Autodesk Inventor part; units mm, degrees
ref_plane "YZ Plane" through (0, 0, 0) normal (1, 0, 0) x (0, 1, 0)
ref_plane "XZ Plane" through (0, 0, 0) normal (0, 1, 0) x (-1, 0, 0)
ref_plane "XY Plane" through (0, 0, 0) normal (0, 0, 1) x (1, 0, 0)
sketch "Boceto1" plane through (0, 0, 0) normal (1, 0, 0) x (0, 1, 0)
  line L0 (25, 5.601225) -> (19, 5.601225)
  line L1 (19, 5.601225) -> (19, -18.398775)
  line L2 (19, -18.398775) -> (15, -18.398775)
  line L3 (15, -18.398775) -> (15, -80.798775)
  line L4 (15, -80.798775) -> (45, -80.798775)
  line L5 (45, -80.798775) -> (45, -68.598775)
  line L6 (45, -68.598775) -> (20, -68.598775)
  line L7 (20, -68.598775) -> (20, -24.398775)
  line L8 (20, -24.398775) -> (25, -24.398775)
  line L9 (25, -24.398775) -> (25, 5.601225)
  line L10 (0, 0) -> (0, 11.507163) construction
  line L11 (-25, 5.601225) -> (-19, 5.601225)
  line L12 (-19, 5.601225) -> (-19, -18.398775)
  line L13 (-19, -18.398775) -> (-15, -18.398775)
  line L14 (-15, -18.398775) -> (-15, -80.798775)
  line L15 (-15, -80.798775) -> (-45, -80.798775)
  line L16 (-45, -80.798775) -> (-45, -68.598775)
  line L17 (-45, -68.598775) -> (-20, -68.598775)
  line L18 (-20, -68.598775) -> (-20, -24.398775)
  line L19 (-20, -24.398775) -> (-25, -24.398775)
  line L20 (-25, -24.398775) -> (-25, 5.601225)
  dimension "d0" = 30
  dimension "d1" = 40
  dimension "d2" = 90
  dimension "d3" = 38
  dimension "d4" = 50
  dimension "d5" = 24
  dimension "d6" = 6
  dimension "d7" = 44.2
  dimension "d8" = 12.2
sketch "Boceto1 outline for Revolución1" plane through (0, 0, 0) normal (1, 0, 0) x (0, 1, 0)
  line L0 (-25, 5.601225) -> (-25, -24.398775)
  line L1 (-19, 5.601225) -> (-25, 5.601225)
  line L2 (-19, -18.398775) -> (-19, 5.601225)
  line L3 (-15, -18.398775) -> (-19, -18.398775)
  line L4 (-15, -80.798775) -> (-15, -18.398775)
  line L5 (-45, -80.798775) -> (-15, -80.798775)
  line L6 (-45, -68.598775) -> (-45, -80.798775)
  line L7 (-20, -68.598775) -> (-45, -68.598775)
  line L8 (-20, -24.398775) -> (-20, -68.598775)
  line L9 (-25, -24.398775) -> (-20, -24.398775)
  line L10 (25, 5.601225) -> (19, 5.601225)
  line L11 (25, -24.398775) -> (25, 5.601225)
  line L12 (20, -24.398775) -> (25, -24.398775)
  line L13 (20, -68.598775) -> (20, -24.398775)
  line L14 (45, -68.598775) -> (20, -68.598775)
  line L15 (45, -80.798775) -> (45, -68.598775)
  line L16 (15, -80.798775) -> (45, -80.798775)
  line L17 (15, -18.398775) -> (15, -80.798775)
  line L18 (19, -18.398775) -> (15, -18.398775)
  line L19 (19, 5.601225) -> (19, -18.398775)
revolve "Revolución1" add sketch "Boceto1 outline for Revolución1" angle 360 about axis through (0, 0, 0) along (0, 0, 1)
sketch "Boceto4" plane through (0, 0, -68.598775) normal (0, 0, 1) x (1, 0, 0)
  circle A0 centre (0, -32.5) radius 6.25
  circle A1 centre (0, 32.5) radius 6.25
  circle A2 centre (-32.5, 0) radius 6.25
  circle A3 centre (32.5, 0) radius 6.25
  circle A4 centre (0, -32.5) radius 6.25
  circle A5 centre (0, 32.5) radius 6.25
  circle A6 centre (32.5, 0) radius 6.25
  circle A7 centre (-32.5, 0) radius 6.25
  point P0 (0, 0)
  dimension "d18" = 12.5
  dimension "d19" = 12.5
  dimension "d20" = 65
  dimension "d21" = 32.5
  dimension "d24" = 360
sketch "Boceto4 outline for Extrusión1" plane through (0, 0, -68.598775) normal (0, 0, 1) x (1, 0, 0)
  circle A0 centre (-32.5, 0) radius 6.25
  circle A1 centre (0, -32.5) radius 6.25
  circle A2 centre (32.5, 0) radius 6.25
  circle A3 centre (0, 32.5) radius 6.25
extrude "Extrusión1" cut sketch "Boceto4 outline for Extrusión1" against normal through all
chamfer "Chaflán1" distance 3 distance2 3.5 1 edges at (0, 15, -80.7988) measured on face at (2.4062, -14.8058, -59.9988)
fillet "Empalme1" radius 2 4 edges at (0, 45, -68.5988) (0, 20, -68.5988) (0, 25, 5.6012) (0, 19, 5.6012)
properties part number "Pieza de practica 2"
Read the model definition and answer for the solid it produces. Units are mm, in the model's axes. A direction names the side the tool comes from. Round coordinates to 2 decimals unless told otherwise and drop trailing zeros. Write each loop counter-clockwise with the first axis right and the second up, starting at its lowest first coordinate (ties: lowest second). Pieces come first, ordered by that corner, then holes. Notation, with made-up numbers: (61.25, 56.25) -> (86.25, 56.25) arc R22 ccw to (86.25, 94.25) -> close; hole circle Ø1 at (37, -37). An arc over 180 degrees is marked (long way). Answer in a Markdown table with one row per item. Add a question column.
1) Find section B-B, the plane z = -26. Determine the outline of the cut face in (x, y), and give its area (3 significant figures).
2) Find section A-A, the plane z = -8.5. Determine the outline of the cut face in (x, y), and give its area (3 significant figures).
3) Consider line 1 (Y direction, x = 0, z = -72); line 2 (X direction, y = 0, z = -55); line 3 (Z direction, x = -21.5, y = -25.5). Determine where each line is inside the solid, lowest interval first.
4) Given P1, Ø10, axis at x = 32.5, y = 0, coming from the +Z side; P2, Ø16, axis at x = 0, y = 32.5, coming from the +Z side; P3, Ø12, axis at x = -14.5, z = -61.5, coming from the -Y side; P4, Ø4, axis at y = 18, z = -68, coming from the -X side, each flat-ended and moving along its own axis, determine where each tip first touches the part or whether it passes through.
5) Determine the mould class of faces 1 (the face through (-19, -10, 5.601)), 2 (the face through (-38.744, 0.275, -74.613)), 3 (the face through (19.524, 4.336, -45.794)), 4 (the face through (-16.856, -8.767, -7.245)) for opening direction X: pulls with the +X half, pulls with the -X half, needs draft (parallel to the pull), parting line crosses it, or undercut.
6) Which of the six approach directions +Z, -Z, +X, -X, +Y, -Y give full straight-line access (tool end or side, diameter ignored) to faces 5 (the face through (17, 11, -24.399)), 6 (the face through (-19, 1, -80.799)), 7 (the face through (6, -14, -18.399))?
Findings below:
| question | item | result |
|---|---|---|
| 1 | outline | circle Ø40 at (0, 0); hole circle Ø30 at (0, 0) |
| 1 | area | 550 mm² |
| 2 | outline | circle Ø50 at (0, 0); hole circle Ø38 at (0, 0) |
| 2 | area | 829 mm² |
| 3 | line 1 | -45 to -38.75, -26.25 to -15, 15 to 26.25, 38.75 to 45 |
| 3 | line 2 | -20 to -15, 15 to 20 |
| 3 | line 3 | -80.8 to -68.6 |
| 4 | P1 | through |
| 4 | P2 | z = 4.92 |
| 4 | P3 | y = -18.1 |
| 4 | P4 | x = -41.46 |
| 5 | face 1 | needs draft |
| 5 | face 2 | undercut |
| 5 | face 3 | parting line crosses it |
| 5 | face 4 | undercut |
| 6 | face 5 | none |
| 6 | face 6 | -Z, +X, -X, +Y, -Y |
| 6 | face 7 | +Z |
